Geometry check sheet. Reference: the model listing, model coordinates, mm. Face numbers are marked on the shaded views. Round coordinates to 2 decimals unless told otherwise and drop trailing zeros. Write each loop counter-clockwise with the first axis right and the second up, starting at its lowest first coordinate (ties: lowest second). Pieces come first, ordered by that corner, then holes.
from build123d import *

# Parameters (mm, degrees)
SKETCH2_W            = 5
SKETCH2_H            = 4
PACKAGE_DEPTH        = 1.5
DRAFT1_START         = -2.5
DRAFT1_DEPTH         = 5
DRAFT1_START_2       = -3
DRAFT1_2_DEPTH       = 6
DRAFT2_START         = -2
DRAFT2_DEPTH         = 4
DRAFT2_START_2       = -3
DRAFT2_2_DEPTH       = 6
CHAMFER1_SIZE        = 0.25
CHAMFER1_SIZE2       = 0.275015717
LEADS_DEPTH          = 0.2
FILLET1_R            = 0.25
FILLET2_R            = 0.125
FILLET1_OF_MIRROR1_R = 0.25
FILLET2_OF_MIRROR1_R = 0.125
LPATTERN1_START      = -0.835
LPATTERN1_DEPTH      = 0.4
LPATTERN1_START_2    = 0.435
LPATTERN1_2_DEPTH    = 0.4
LPATTERN1_START_3    = 1.705
LPATTERN1_3_DEPTH    = 0.4
SKETCH4_R            = 0.225
MARKER_DEPTH         = 0.1


with BuildPart() as part:
    # Sketch2 → Package (new body)
    with BuildSketch(Plane(origin=(0, 0.25, 0), x_dir=(-1, 0, 0), z_dir=(0, 1, 0))):
        Rectangle(SKETCH2_W, SKETCH2_H)
    extrude(amount=PACKAGE_DEPTH)

    # Draft1: read off the stored shape, not the designer's step
    # Draft1 outline → Draft1 (cut)
    with BuildSketch(Plane.YZ.offset(DRAFT1_START)):
        Polygon((1.75, -2), (1.75, -1.934383502), (1, -2), align=None)
        Polygon((1, 2), (1.75, 1.934383502), (1.75, 2), align=None)
    extrude(amount=DRAFT1_DEPTH, mode=Mode.SUBTRACT)

    # Draft1 2 outline → Draft1 2 (cut)
    with BuildSketch(Plane.XY.offset(DRAFT1_START_2)):
        Polygon((-2.5, 1), (-2.434383502, 1.75), (-2.5, 1.75), align=None)
        Polygon((2.434383502, 1.75), (2.5, 1), (2.5, 1.75), align=None)
    extrude(amount=DRAFT1_2_DEPTH, mode=Mode.SUBTRACT)

    # Draft2: read off the stored shape, not the designer's step
    # Draft2 outline → Draft2 (cut)
    with BuildSketch(Plane.XY.offset(DRAFT2_START)):
        Polygon((2.5, 0.75), (2.456255668, 0.25), (2.5, 0.25), align=None)
        Polygon((-2.456255668, 0.25), (-2.5, 0.75), (-2.5, 0.25), align=None)
    extrude(amount=DRAFT2_DEPTH, mode=Mode.SUBTRACT)

    # Draft2 2 outline → Draft2 2 (cut)
    with BuildSketch(Plane.YZ.offset(DRAFT2_START_2)):
        Polygon((0.75, -2), (0.25, -1.956255668), (0.25, -2), align=None)
        Polygon((0.25, 1.956255668), (0.75, 2), (0.25, 2), align=None)
    extrude(amount=DRAFT2_2_DEPTH, mode=Mode.SUBTRACT)

    # Chamfer1
    chamfer1_edges = [part.edges().sort_by_distance(p)[0] for p in [
        (0, 1.75, 1.934383502),
    ]]
    chamfer1_side = [part.faces().sort_by_distance(p)[0] for p in [
        (0, 1.373337774, 1.967337177),
    ]]
    chamfer(chamfer1_edges, length=CHAMFER1_SIZE, length2=CHAMFER1_SIZE2, reference=chamfer1_side[0])

    # Sketch3 → Leads (add, symmetric)
    with BuildSketch(Plane.ZY.offset(1.905)):
        Polygon((-2, 1), (-2, 0.75), (2.5, 0.75), (2.5, 0), (3.1, 0), (3.1, 0.25), (2.75, 0.25), (2.75, 1), align=None)
    leads = extrude(amount=LEADS_DEPTH, both=True)

    # Fillet1
    fillet1_edges = [part.edges().sort_by_distance(p)[0] for p in [
        (-1.905, 1, 2.75),
        (-1.905, 0, 2.5),
    ]]
    fillet(fillet1_edges, radius=FILLET1_R)

    # Fillet2
    fillet2_edges = [part.edges().sort_by_distance(p)[0] for p in [
        (-1.905, 0.75, 2.5),
        (-1.905, 0.25, 2.75),
    ]]
    fillet(fillet2_edges, radius=FILLET2_R)

    # Mirror1: Leads across plane
    add(leads.mirror(Plane.XY))

    # Fillet1 of Mirror1
    fillet1_of_mirror1_edges = [part.edges().sort_by_distance(p)[0] for p in [
        (-1.905, 1, -2.75),
        (-1.905, 0, -2.5),
    ]]
    fillet(fillet1_of_mirror1_edges, radius=FILLET1_OF_MIRROR1_R)

    # Fillet2 of Mirror1
    fillet2_of_mirror1_edges = [part.edges().sort_by_distance(p)[0] for p in [
        (-1.905, 0.75, -2.5),
        (-1.905, 0.25, -2.75),
    ]]
    fillet(fillet2_of_mirror1_edges, radius=FILLET2_OF_MIRROR1_R)

    # LPattern1: read off the stored shape, not the designer's step
    # LPattern1 outline → LPattern1 (add)
    with BuildSketch(Plane.YZ.offset(LPATTERN1_START)):
        with BuildLine():
            Line((1, 2), (1, 2.5))
            ThreePointArc((1, 2.5), (0.926776695, 2.676776695), (0.75, 2.75))
            Line((0.75, 2.75), (0.375, 2.75))
            ThreePointArc((0.375, 2.75), (0.286611652, 2.786611652), (0.25, 2.875))
            Line((0.25, 2.875), (0.25, 3.1))
            Line((0.25, 3.1), (0, 3.1))
            Line((0, 3.1), (0, 2.75))
            ThreePointArc((0, 2.75), (0.073223305, 2.573223305), (0.25, 2.5))
            Line((0.25, 2.5), (0.625, 2.5))
            ThreePointArc((0.625, 2.5), (0.713388348, 2.463388348), (0.75, 2.375))
            Line((0.75, 2.375), (0.75, 2))
            Line((0.75, 2), (1, 2))
        make_face()
        with BuildLine():
            ThreePointArc((0.75, -2.75), (0.926776695, -2.676776695), (1, -2.5))
            Line((1, -2.5), (1, -2))
            Line((1, -2), (0.75, -2))
            Line((0.75, -2), (0.75, -2.375))
            ThreePointArc((0.75, -2.375), (0.713388348, -2.463388348), (0.625, -2.5))
            Line((0.625, -2.5), (0.25, -2.5))
            ThreePointArc((0.25, -2.5), (0.073223305, -2.573223305), (0, -2.75))
            Line((0, -2.75), (0, -3.1))
            Line((0, -3.1), (0.25, -3.1))
            Line((0.25, -3.1), (0.25, -2.875))
            ThreePointArc((0.25, -2.875), (0.286611652, -2.786611652), (0.375, -2.75))
            Line((0.375, -2.75), (0.75, -2.75))
        make_face()
    extrude(amount=LPATTERN1_DEPTH)

    # LPattern1 2 outline → LPattern1 2 (add)
    with BuildSketch(Plane.YZ.offset(LPATTERN1_START_2)):
        with BuildLine():
            Line((1, 2), (1, 2.5))
            ThreePointArc((1, 2.5), (0.926776695, 2.676776695), (0.75, 2.75))
            Line((0.75, 2.75), (0.375, 2.75))
            ThreePointArc((0.375, 2.75), (0.286611652, 2.786611652), (0.25, 2.875))
            Line((0.25, 2.875), (0.25, 3.1))
            Line((0.25, 3.1), (0, 3.1))
            Line((0, 3.1), (0, 2.75))
            ThreePointArc((0, 2.75), (0.073223305, 2.573223305), (0.25, 2.5))
            Line((0.25, 2.5), (0.625, 2.5))
            ThreePointArc((0.625, 2.5), (0.713388348, 2.463388348), (0.75, 2.375))
            Line((0.75, 2.375), (0.75, 2))
            Line((0.75, 2), (1, 2))
        make_face()
        with BuildLine():
            ThreePointArc((0.75, -2.75), (0.926776695, -2.676776695), (1, -2.5))
            Line((1, -2.5), (1, -2))
            Line((1, -2), (0.75, -2))
            Line((0.75, -2), (0.75, -2.375))
            ThreePointArc((0.75, -2.375), (0.713388348, -2.463388348), (0.625, -2.5))
            Line((0.625, -2.5), (0.25, -2.5))
            ThreePointArc((0.25, -2.5), (0.073223305, -2.573223305), (0, -2.75))
            Line((0, -2.75), (0, -3.1))
            Line((0, -3.1), (0.25, -3.1))
            Line((0.25, -3.1), (0.25, -2.875))
            ThreePointArc((0.25, -2.875), (0.286611652, -2.786611652), (0.375, -2.75))
            Line((0.375, -2.75), (0.75, -2.75))
        make_face()
    extrude(amount=LPATTERN1_2_DEPTH)

    # LPattern1 3 outline → LPattern1 3 (add)
    with BuildSketch(Plane.YZ.offset(LPATTERN1_START_3)):
        with BuildLine():
            Line((1, 2), (1, 2.5))
            ThreePointArc((1, 2.5), (0.926776695, 2.676776695), (0.75, 2.75))
            Line((0.75, 2.75), (0.375, 2.75))
            ThreePointArc((0.375, 2.75), (0.286611652, 2.786611652), (0.25, 2.875))
            Line((0.25, 2.875), (0.25, 3.1))
            Line((0.25, 3.1), (0, 3.1))
            Line((0, 3.1), (0, 2.75))
            ThreePointArc((0, 2.75), (0.073223305, 2.573223305), (0.25, 2.5))
            Line((0.25, 2.5), (0.625, 2.5))
            ThreePointArc((0.625, 2.5), (0.713388348, 2.463388348), (0.75, 2.375))
            Line((0.75, 2.375), (0.75, 2))
            Line((0.75, 2), (1, 2))
        make_face()
        with BuildLine():
            ThreePointArc((0.75, -2.75), (0.926776695, -2.676776695), (1, -2.5))
            Line((1, -2.5), (1, -2))
            Line((1, -2), (0.75, -2))
            Line((0.75, -2), (0.75, -2.375))
            ThreePointArc((0.75, -2.375), (0.713388348, -2.463388348), (0.625, -2.5))
            Line((0.625, -2.5), (0.25, -2.5))
            ThreePointArc((0.25, -2.5), (0.073223305, -2.573223305), (0, -2.75))
            Line((0, -2.75), (0, -3.1))
            Line((0, -3.1), (0.25, -3.1))
            Line((0.25, -3.1), (0.25, -2.875))
            ThreePointArc((0.25, -2.875), (0.286611652, -2.786611652), (0.375, -2.75))
            Line((0.375, -2.75), (0.75, -2.75))
        make_face()
    extrude(amount=LPATTERN1_3_DEPTH)

    # Sketch4 → Marker (cut)
    with BuildSketch(Plane(origin=(0, 1.75, 0), x_dir=(1, 0, 0), z_dir=(0, 1, 0))):
        with Locations(Location((-1.905, -1.2, 0), (0, 0, 270))):
            Circle(SKETCH4_R)
    extrude(amount=-MARKER_DEPTH, mode=Mode.SUBTRACT)


solid = part.part
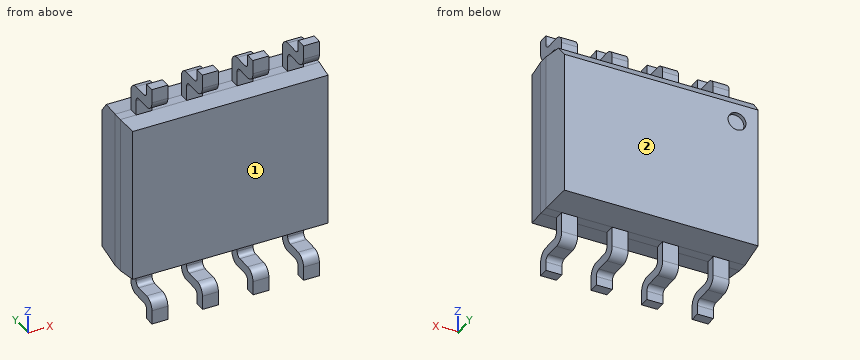
1. Section check A-A (z = 1.2). Record the cut outline in (x, y).
2. Depth check by flat-ended pin: pin 1 Ø2 at (x, z) = (0, 0) entering from -Y; pin 2 Ø0.5 at (y, z) = (0.5, 2.5) entering from -X (3 decimals). Enter the tip coordinate at first touch or a pass-through.
3. Section check C-C (y = 0.55). State how many separate pieces and enclosed holes the cut face has, plus the area to 3 significant figures.
4. Release check for a two-part mould opening along Z. For the marked faces 1 and 2 record: +Z half, -Z half, draft (parallel to the pull), parting line (faces both ways), or undercut.
5. Section check B-B (x = 1.1). Record the cut outline in (y, z).
6. Scan lines: line 1 along X through (y, z) = (0.9, -2.5) (3 decimals); line 2 along Z through (x, y) = (-0.5, 0.5); line 3 along Y through (x, z) = (0.7, -1.5). Record each from-to range of solid material in increasing order.
7. Section check D-D (z = -0.75). Record the cut outline in (x, y).
Results below:
1. outline: (-2.5, 0.75) - (-2.46, 0.25) - (2.46, 0.25) - (2.5, 0.75) - (2.5, 1) - (2.43, 1.75) - (-1.68, 1.75) - (-1.68, 1.65) - (-2.13, 1.65) - (-2.13, 1.75) - (-2.43, 1.75) - (-2.5, 1) - close
2. pin 1: stops at y = 0.25
2. pin 2: stops at x = -2.105
3. separate pieces: 9
3. enclosed holes: 0
3. area: 20.5 mm2
4. face 1: undercut
4. face 2: draft
5. outline: (0.25, -1.96) - (0.75, -2) - (1, -2) - (1.75, -1.93) - (1.75, 1.66) - (1.5, 1.96) - (1, 2) - (0.75, 2) - (0.25, 1.96) - close
6. line 1: x = -2.105 to -1.705, -0.835 to -0.435, 0.435 to 0.835, 1.705 to 2.105
6. line 2: z = -2.75 to -2.5, -1.98 to 1.98, 2.5 to 2.75
6. line 3: y = 0.25 to 1.75
7. outline: (-2.5, 0.75) - (-2.46, 0.25) - (2.46, 0.25) - (2.5, 0.75) - (2.5, 1) - (2.43, 1.75) - (-2.43, 1.75) - (-2.5, 1) - close
